```python
from build123d import *

# Parameters (mm, degrees)
SKETCH1_R                 = 18.85
BOSS_EXTRUDE1_DEPTH       = 28.5
SKETCH2_R                 = 2
BOSS_EXTRUDE2_DEPTH       = 6
SKETCH3_R                 = 2
BOSS_EXTRUDE3_DEPTH       = 2.6
M3X0_5_TAPPED_HOLE1_D     = 2.5
M3X0_5_TAPPED_HOLE1_DEPTH = 1.648924226
M3X0_5_TAPPED_HOLE1_TIP   = 0.751075774
M3X0_5_TAPPED_HOLE2_D     = 2.5
M3X0_5_TAPPED_HOLE2_DEPTH = 5.248924226
M3X0_5_TAPPED_HOLE2_TIP   = 0.751075774


with BuildPart() as part:
    # Sketch1 → Boss-Extrude1 (new body)
    with BuildSketch(Plane(origin=(0, 0, 0), x_dir=(1, 0, 0), z_dir=(0, 1, 0))):
        Circle(SKETCH1_R)
    extrude(amount=BOSS_EXTRUDE1_DEPTH)

    # Sketch2 → Boss-Extrude2 (add)
    with BuildSketch(Plane(origin=(0, 28.5, 0), x_dir=(1, 0, 0), z_dir=(0, 1, 0))):
        Circle(SKETCH2_R)
    extrude(amount=BOSS_EXTRUDE2_DEPTH)

    # Sketch3 → Boss-Extrude3 (add)
    with BuildSketch(Plane.XZ):
        Circle(SKETCH3_R)
    extrude(amount=BOSS_EXTRUDE3_DEPTH)

    # M3x0.5 Tapped Hole1
    with Locations(Plane(origin=(0, 0, 9.5), x_dir=(0, 0, -1), z_dir=(0, -1, 0))):
        with Locations((0, 0), (9.5, 8), (9.5, 12.5), (19, 0), (9.5, -8), (9.5, -12.5)):
            Hole(M3X0_5_TAPPED_HOLE1_D / 2, depth=M3X0_5_TAPPED_HOLE1_DEPTH)
            with Locations((0, 0, -(M3X0_5_TAPPED_HOLE1_DEPTH + M3X0_5_TAPPED_HOLE1_TIP / 2))):  # 118° drill point
                Cone(0, M3X0_5_TAPPED_HOLE1_D / 2, M3X0_5_TAPPED_HOLE1_TIP, mode=Mode.SUBTRACT)

    # Sketch10 → Cut-Revolve1 (revolve, cut)
    with BuildSketch(Plane.XY):
        Polygon((-18.85, 28.5), (-10, 28.5), (-18.85, 22.5), align=None)
        with BuildLine():
            Line((-18.85, 2.6), (-18.85, 0))
            Line((-18.85, 0), (-16, 0))
            ThreePointArc((-16, 0), (-16.921107831, 1.852343339), (-18.85, 2.6))
        make_face()
    revolve(axis=Axis((0, 28.5, 0), (0, -1, 0)), mode=Mode.SUBTRACT)

    # M3x0.5 Tapped Hole2
    with Locations(Plane(origin=(0, 28.5, -6), x_dir=(0, 0, 1), z_dir=(0, 1, 0))):
        with Locations((0, 0), (6, 6), (12, 0), (6, -6)):
            Hole(M3X0_5_TAPPED_HOLE2_D / 2, depth=M3X0_5_TAPPED_HOLE2_DEPTH)
            with Locations((0, 0, -(M3X0_5_TAPPED_HOLE2_DEPTH + M3X0_5_TAPPED_HOLE2_TIP / 2))):  # 118° drill point
                Cone(0, M3X0_5_TAPPED_HOLE2_D / 2, M3X0_5_TAPPED_HOLE2_TIP, mode=Mode.SUBTRACT)


solid = part.part
```
Could you check a few things on this model? Use its own coordinates, in mm. A direction names the side the tool comes from. Round coordinates to 2 decimals unless told otherwise and drop trailing zeros. Loops run counter-clockwise (first coordinate to the right, second up) from the corner with the lowest first, then second, coordinate; pieces in that order, holes last. Notation, with made-up numbers: (-27.5, -1.75) - (8.5, -1.75) arc R26 ccw to (8.5, 33.25) - close; hole circle Ø7 at (70.5, 78). An arc over 180 degrees is marked (long way). Answer in a Markdown table with one row per item. Add a question column.
(1) For faces 4 (the face through (-7.22, 25.84, 0.27)), 5 (the face through (-9.22, 0.84, -0.27)), which set-ups out of +Z, -Z, +X, -X, +Y, -Y let a thin tool reach every point of the face, with its end or its side?
(2) I'm going to push flat-ended pins straight in: pin 1 (4 mm diameter, centred on x = 0, z = 6, fed in from -Y); pin 2 (6 mm diameter, centred on y = 23, z = 11.5, fed in from -X); pin 3 (2 mm diameter, centred on x = -6, z = 0, fed in from +Y). Where does each tip first touch, or does it pass through?
(3) I need wall thicknesses on line 1 along Z through (x, y) = (1, 27); line 2 along Z through (x, y) = (0, 0.8); line 3 along Z through (x, y) = (-8, 1). Which ranges of each line are inside material? Lowest first, please.
(4) If we section it at A-A (y = 1): Please give me the cut outline in (x, z).
(5) If we mould it in two halves opening along Z, with no side actions, what happens to faces 1 (the face through (3, 0, 0)), 2 (the face through (-4.1, 12.4, 18.4)), 3 (the face through (-0.08, 2.27, -9.7))? For each: pulls with the +Z half, pulls with the -Z half, needs draft (parallel to the pull), parting line crosses it, or undercut.
Model answer:
| question | item | result |
|---|---|---|
| 1 | face 4 | +Y |
| 1 | face 5 | -Y |
| 2 | pin 1 | stops at y = 0 |
| 2 | pin 2 | stops at x = -16.8 |
| 2 | pin 3 | stops at y = 23.1 |
| 3 | line 1 | z = -12.17 to -6.75, -5.25 to 5.25, 6.75 to 12.17 |
| 3 | line 2 | z = -16.19 to -10.75, -8.25 to 8.25, 10.75 to 16.19 |
| 3 | line 3 | z = -14.18 to -1.25, 1.25 to 14.18 |
| 4 | outline | circle Ø32.56 at (0, 0); hole circle Ø2.5 at (-12.5, 0); hole circle Ø2.5 at (-8, 0); hole circle Ø2.5 at (0, -9.5); hole circle Ø2.5 at (0, 9.5); hole circle Ø2.5 at (8, 0); hole circle Ø2.5 at (12.5, 0) |
| 5 | face 1 | needs draft |
| 5 | face 2 | parting line crosses it |
| 5 | face 3 | undercut |
